The model under review builds one solid part; all positions refer to its coordinate system, in mm. A direction names the side the tool comes from. Round coordinates to 2 decimals unless told otherwise and drop trailing zeros. Order: outer loops, then holes, each group sorted by start corner. A loop starts at its lowest first (then second) coordinate and runs counter-clockwise, first axis right, second up. Notation, with made-up numbers: (39.5, 56) -> (62.5, 56) arc R17 cw to (62.5, 75) -> close; hole circle Ø3 at (82.5, 83). An arc over 180 degrees is marked (long way). Return JSON: item names as keys, results as strings. Group by question number.
Autodesk Inventor part; units mm, degrees
ref_plane "YZ Plane" through (0, 0, 0) normal (1, 0, 0) x (0, 1, 0)
ref_plane "XZ Plane" through (0, 0, 0) normal (0, 1, 0) x (-1, 0, 0)
ref_plane "XY Plane" through (0, 0, 0) normal (0, 0, 1) x (1, 0, 0)
sketch "Sketch1" plane through (0, 0, 0) normal (0, 0, 1) x (1, 0, 0)
  ellipse E0 centre (0, 0) end of major axis (0, 70) minor radius 61.5 construction
  line L0 (-6.6, -55) -> (6.6, -55) construction
  line L1 (6.6, -55) -> (6.6, -63.55) construction
  line L2 (6.6, -63.55) -> (-6.6, -63.55) construction
  line L3 (-6.6, -63.55) -> (-6.6, -55) construction
  line L4 (0, 0) -> (0, -55) construction
  line L5 (-6.75, -54.5) -> (6.75, -54.5)
  line L6 (6.75, -54.5) -> (6.75, -64.05)
  line L7 (6.75, -64.05) -> (-6.75, -64.05)
  line L8 (-6.75, -64.05) -> (-6.75, -54.5)
  line L9 (9, -53.775) -> (-9, -53.775)
  line L10 (-9, -53.775) -> (-9, -64.775)
  line L11 (-9, -64.775) -> (9, -64.775)
  line L12 (9, -64.775) -> (9, -53.775)
  line L13 (6.75, -59.275) -> (-6.75, -59.275) construction
  line L14 (9, -53.775) -> (15, -53.775)
  line L15 (15, -53.775) -> (15, -56.275)
  line L16 (15, -56.275) -> (9, -56.275)
  line L17 (9, -56.275) -> (9, -53.775)
  line L18 (-9, -53.775) -> (-15, -53.775)
  line L19 (-15, -53.775) -> (-15, -56.275)
  line L20 (-15, -56.275) -> (-9, -56.275)
  dimension "d0" = 8.55
  dimension "d1" = 13.2
  dimension "d2" = 55
  dimension "d3" = 0.5
  dimension "d4" = 0.5
  dimension "d5" = 13.5
  dimension "d6" = 6.75
  dimension "d7" = 18
  dimension "d8" = 9
  dimension "d9" = 11
  dimension "d10" = 5.5
  dimension "d20" = 2.5
  dimension "d21" = 6
extrude "Extrusion1" add sketch "Sketch1" against normal blind 15.6
sketch "Sketch2" plane through (0, 0, 0) normal (0, 0, 1) x (1, 0, 0)
  line L0 (-9, -56.275) -> (-9, -64.775)
  line L1 (-9, -64.775) -> (9, -64.775)
  line L2 (9, -64.775) -> (9, -56.275)
  line L3 (-6.75, -54.5) -> (6.75, -54.5)
  line L4 (6.75, -54.5) -> (6.75, -64.05)
  line L5 (6.75, -64.05) -> (-6.75, -64.05)
  line L6 (-6.75, -64.05) -> (-6.75, -54.5)
  line L7 (6.75, -54.5) -> (7.5, -54.5)
  line L8 (7.5, -54.5) -> (7.5, -64.05)
  line L9 (7.5, -64.05) -> (6.75, -64.05)
  line L10 (6.75, -64.05) -> (6.75, -54.5)
  line L11 (-6.75, -54.5) -> (-7.5, -54.5)
  line L12 (-7.5, -54.5) -> (-7.5, -64.05)
  line L13 (-7.5, -64.05) -> (-6.75, -64.05)
  line L14 (-6.75, -64.05) -> (-6.75, -54.5)
  line L15 (6.75, -64.05) -> (-6.75, -64.05)
  line L16 (9, -56.275) -> (15, -56.275)
  line L17 (15, -56.275) -> (15, -53.775)
  line L18 (15, -53.775) -> (-15, -53.775)
  line L19 (-15, -53.775) -> (-15, -56.275)
  line L20 (-15, -56.275) -> (-9, -56.275)
  point P0 (0, 0)
  dimension "d13" = 0.75
  dimension "d14" = 0.75
extrude "Extrusion2" cut sketch "Sketch2" against normal blind 13.6 contours L6 L13 L12 L11 | L7 L8 L9 L4
chamfer "Chamfer1" distance 0.75 angle 45 2 edges at (7.5, -59.275, -13.6) (-7.5, -59.275, -13.6)
fillet "Fillet1" radius 4 4 edges at (15, -55.025, -15.6) (15, -55.025, 0) (-15, -55.025, 0) (-15, -55.025, -15.6)
chamfer "Chamfer2" distance 0.75 angle 45 2 edges at (9, -56.275, -7.8) (-9, -56.275, -7.8)
equation "\"d6\" = 0.5 * d5"
equation "\"d8\" = 0.5 * d7"
equation "\"d10\" = 0.5 * d9"
properties part number "new_power_switch"
Item 1: Consider section C-C on z = -10.75. State the section outline as (x, y) points (3 decimals), plus the area to 3 significant figures.
Item 2: Consider section B-B on x = 5. State the section outline as (y, z) points (3 decimals), plus the area to 3 significant figures.
Item 3: Insertion check: pin 1 Ø1 at (x, y) = (1.5, -62.5) entering from +Z; pin 2 Ø3 at (y, z) = (-61.5, -8.5) entering from +X; pin 3 Ø2.5 at (x, z) = (11.5, -6) entering from -Y (3 decimals); pin 4 Ø3 at (y, z) = (-60, -8) entering from -X. Each pin has a flat end and moves straight along its axis. Give the tip position at first contact, or say it passes through.
Item 4: For faces 1 (the face through (-12, -56.275, -8)), 2 (the face through (-6.75, -59, -15)), 3 (the face through (9, -61, -8)), list the 3-axis set-ups (+Z, -Z, +X, -X, +Y, -Y) from which the entire face can be reached by the end or side of a thin tool; tool diameter is ignored.
Item 5: The part is to be moulded in two halves that separate along X. For faces 4 (the face through (0, -53.775, -8)), 5 (the face through (-13.797, -55.042, -1.141)), 6 (the face through (6.75, -59, -15)), say which applies: +X half, -X half, draft (parallel to the pull), parting line (faces both ways), or undercut.
Item 6: Wall thickness on line 1 along Y through (x, z) = (-7.25, -10.25) (3 decimals); line 2 along X through (y, z) = (-55.75, -4.75); line 3 along X through (y, z) = (-61, -3.25): over which ranges is each line inside the solid? List them lowest first.
Values:
{
 "1": {"outline": "(-15, -56.275) -> (-9.75, -56.275) -> (-9, -57.025) -> (-9, -64.775) -> (9, -64.775) -> (9, -57.025) -> (9.75, -56.275) -> (15, -56.275) -> (15, -53.775) -> (-15, -53.775) -> close; hole (-7.5, -64.05) -> (7.5, -64.05) -> (7.5, -54.5) -> (-7.5, -54.5) -> close", "area": "85.3 mm^2"},
 "2": {"outline": "(-64.775, -15.6) -> (-64.05, -15.6) -> (-64.05, 0) -> (-64.775, 0) -> close; (-54.5, -15.6) -> (-53.775, -15.6) -> (-53.775, 0) -> (-54.5, 0) -> close", "area": "22.6 mm^2"},
 "3": {"pin 1": "through", "pin 2": "x = 9", "pin 3": "y = -56.275", "pin 4": "x = -9"},
 "4": {"face 1": "+Z, -Z, -X, -Y", "face 2": "+Z, -Z", "face 3": "+Z, -Z, +X, -Y"},
 "5": {"face 4": "draft", "face 5": "-X half", "face 6": "undercut"},
 "6": {"line 1": "-64.775 to -64.05, -54.5 to -53.775", "line 2": "-15 to -7.5, 7.5 to 15", "line 3": "-9 to -7.5, 7.5 to 9"}
}
